Geometry: see drawing. Coordinates: mm, zero at the bounding-box minimum. A direction names the side the tool comes from. Round coordinates to 2 decimals unless told otherwise and drop trailing zeros. Write each loop counter-clockwise with the first axis right and the second up, starting at its lowest first coordinate (ties: lowest second). Pieces come first, ordered by that corner, then holes. Notation, with made-up numbers: (-4, 35) -> (55, 35) arc R9 cw to (55, 42) -> close; hole circle Ø6 at (20, 26). An arc over 180 degrees is marked (long way). Use CSV: the item, a comma, the result in double quotes.
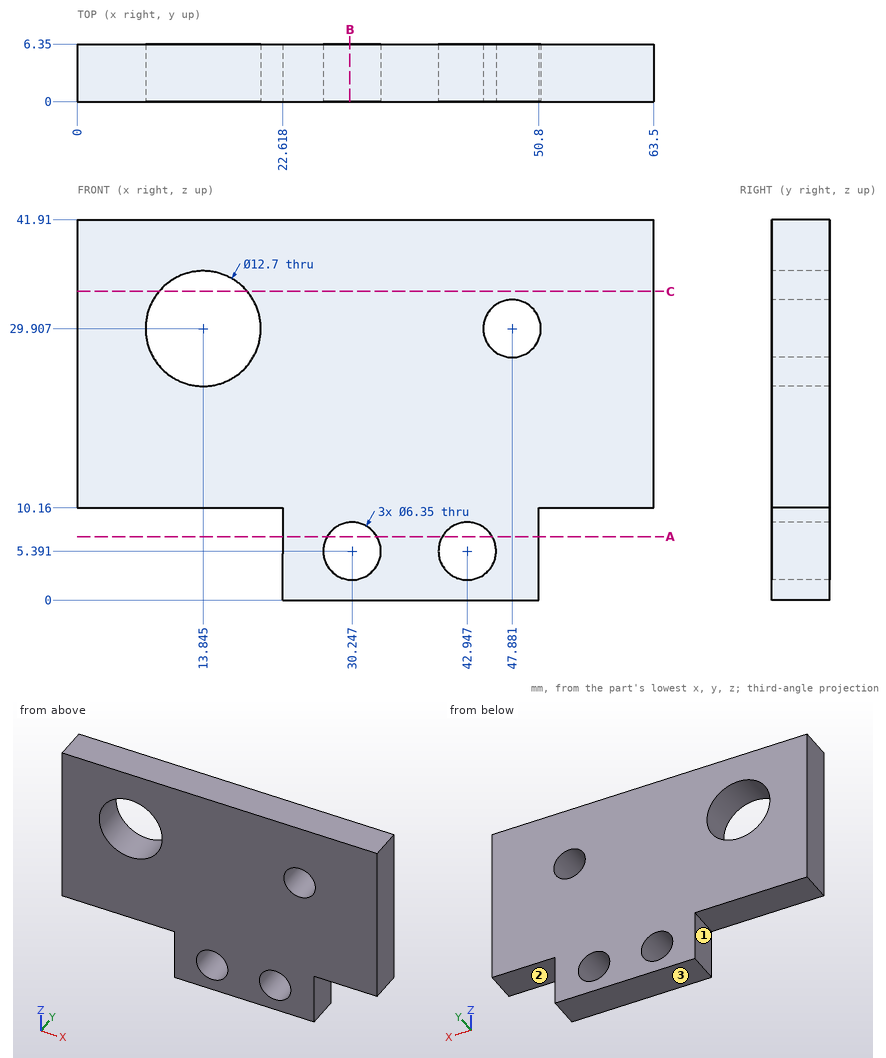
Item 1: Section query A-A on z = 7. Give the number of separate pieces and of enclosed holes in the cut face, plus the area to 3 significant figures.
Worked answers:
separate pieces,"3"
enclosed holes,"0"
area,"109 mm²"
Item 2: Line query: line 1 (X direction, y = 2.5, z = 30) (1 decimal); line 2 (X direction, y = 1, z = 3) (1 decimal); line 3 (Z direction, x = 58.5, y = 6). Output: solid intervals per line, ascending.
Worked answers:
line 1,"x = 0 to 7.5, 20.2 to 44.7, 51.1 to 63.5"
line 2,"x = 22.6 to 28.2, 32.3 to 40.9, 45 to 50.8"
line 3,"z = 10.16 to 41.91"
Item 3: First-contact query: pin 1 Ø5 at (x, z) = (30.25, 5.39) entering from -Y. Flat tip, straight axial feed; report the tip coordinate or a pass-through.
Worked answers:
pin 1,"passes through"
Item 4: Section query B-B on x = 30. Return the cut outline in (y, z).
Worked answers:
outline,"(0, 0) -> (6.35, 0) -> (6.35, 2.23) -> (0, 2.23) -> close; (0, 8.56) -> (6.35, 8.56) -> (6.35, 41.91) -> (0, 41.91) -> close"
Item 5: Set-up query: the marked faces 1, 2 and 3. Return all of +Z, -Z, +X, -X, +Y, -Y with unobstructed straight access to the full face (end or side cutting, diameter ignored); none if empty.
Worked answers:
face 1,"-Z, -X, +Y, -Y"
face 2,"-Z, +X, +Y, -Y"
face 3,"-Z, +X, -X, +Y, -Y"
Item 6: Section query C-C on z = 34. Return the cut outline in (x, y).
Worked answers:
outline,"(0, 0) -> (8.99, 0) -> (8.99, 6.35) -> (0, 6.35) -> close; (18.7, 0) -> (63.5, 0) -> (63.5, 6.35) -> (18.7, 6.35) -> close"
